```python
from build123d import *

# Parameters (mm, degrees)
SKETCH1_W                        = 125
SKETCH1_H                        = 115
TEST_BASE_POSTION_DEPTH          = 9.215
SKETCH8_R                        = 21.5
FINGER_GEARS_DEPTH               = 5
SKETCH9_R                        = 11
INTERMEDIATE_GEAR_DEPTH          = 5
SKETCH11_R                       = 18
XL320_FINGER_KNUCKLE_MOUNT_DEPTH = 5
SKETCH10_R                       = 15.5
CONNECT_FINGER_HOLES_DEPTH       = 86.424915715
THUMB_MOUNT_HOLES_R              = 2
THUMB_MOUNT_HOLES_M4_DEPTH       = 86.424915715
SKETCH16_R                       = 2
FINGERS_MOUNT_HOLES_M4_DEPTH     = 86.424915715
SKETCH17_R                       = 2.8
CONNECT_HOLES_M6_DEPTH           = 86.424915715
SKETCH18_R                       = 3.75
NUTS_M4_DEPTH                    = 4
SKETCH19_R                       = 5.25
CUT_EXTRUDE5_DEPTH               = 6


with BuildPart() as part:
    # Sketch1 → Test_Base_Postion (new body)
    with BuildSketch(Plane(origin=(0, 0, 0), x_dir=(1, 0, 0), z_dir=(0, 1, 0))):
        Rectangle(SKETCH1_W, SKETCH1_H)
    extrude(amount=TEST_BASE_POSTION_DEPTH)

    # Sketch8 → Finger_Gears (cut)
    with BuildSketch(Plane(origin=(0, 9.215, 0), x_dir=(1, 0, 0), z_dir=(0, 1, 0))):
        with Locations((-32.5, -19)):
            Circle(SKETCH8_R)
        with Locations((-32.5, 19)):
            Circle(SKETCH8_R)
    extrude(amount=-FINGER_GEARS_DEPTH, mode=Mode.SUBTRACT)

    # Sketch9 → Intermediate_Gear (cut)
    with BuildSketch(Plane(origin=(0, 9.215, 0), x_dir=(1, 0, 0), z_dir=(0, 1, 0))):
        with Locations((-8.576859648, -4.450657895)):
            Circle(SKETCH9_R)
    extrude(amount=-INTERMEDIATE_GEAR_DEPTH, mode=Mode.SUBTRACT)

    # Sketch11 → XL320_Finger_Knuckle_Mount (cut)
    with BuildSketch(Plane(origin=(0, 9.215, 0), x_dir=(1, 0, 0), z_dir=(0, 1, 0))):
        with Locations(Location((42, 0, 0), (0, 0, 270))):
            Circle(SKETCH11_R)
    extrude(amount=-XL320_FINGER_KNUCKLE_MOUNT_DEPTH, mode=Mode.SUBTRACT)

    # Sketch10 → Connect_Finger_Holes (cut, through all)
    with BuildSketch(Plane(origin=(0, 9.215, 0), x_dir=(1, 0, 0), z_dir=(0, 1, 0))):
        with Locations(Location((-32.5, 19, 0), (0, 0, 270))):
            Circle(SKETCH10_R)
        with Locations(Location((-32.5, -19, 0), (0, 0, 270))):
            Circle(SKETCH10_R)
        with Locations(Location((42, 0, 0), (0, 0, 270))):
            Circle(SKETCH10_R)
    extrude(amount=-CONNECT_FINGER_HOLES_DEPTH, mode=Mode.SUBTRACT)

    # Thumb_Mount_Holes → Thumb_Mount_Holes_(M4) (cut, through all)
    with BuildSketch(Plane(origin=(0, 9.215, 0), x_dir=(1, 0, 0), z_dir=(0, 1, 0))):
        with Locations(Location((22.5, 45.5, 0), (0, 0, 270))):
            Circle(THUMB_MOUNT_HOLES_R)
        with Locations(Location((42, 52.5, 0), (0, 0, 270))):
            Circle(THUMB_MOUNT_HOLES_R)
        with Locations(Location((48, -24, 0), (0, 0, 270))):
            Circle(THUMB_MOUNT_HOLES_R)
        with Locations(Location((36, -24, 0), (0, 0, 90))):
            Circle(THUMB_MOUNT_HOLES_R)
    extrude(amount=-THUMB_MOUNT_HOLES_M4_DEPTH, mode=Mode.SUBTRACT)

    # Sketch16 → Fingers_Mount_Holes_(M4) (cut, through all)
    with BuildSketch(Plane(origin=(0, 9.215, 0), x_dir=(1, 0, 0), z_dir=(0, 1, 0))):
        with Locations(Location((5.25, 38.5, 0), (0, 0, 270))):
            Circle(SKETCH16_R)
        with Locations(Location((5.25, -38.5, 0), (0, 0, 90))):
            Circle(SKETCH16_R)
    extrude(amount=-FINGERS_MOUNT_HOLES_M4_DEPTH, mode=Mode.SUBTRACT)

    # Sketch17 → Connect_Holes_(M6) (cut, through all)
    with BuildSketch(Plane(origin=(0, 9.215, 0), x_dir=(1, 0, 0), z_dir=(0, 1, 0))):
        with Locations(Location((-52.5, 47.5, 0), (0, 0, 270))):
            Circle(SKETCH17_R)
        with Locations(Location((-52.5, -47.5, 0), (0, 0, 90))):
            Circle(SKETCH17_R)
        with Locations(Location((52.5, -47.5, 0), (0, 0, 270))):
            Circle(SKETCH17_R)
    extrude(amount=-CONNECT_HOLES_M6_DEPTH, mode=Mode.SUBTRACT)

    # Sketch18 → Nuts_(M4) (cut)
    with BuildSketch(Plane.XZ):
        with Locations(Location((5.25, 38.5, 0), (0, 0, 270))):
            Circle(SKETCH18_R)
        with Locations(Location((5.25, -38.5, 0), (0, 0, 270))):
            Circle(SKETCH18_R)
        with Locations(Location((22.5, -45.5, 0), (0, 0, 270))):
            Circle(SKETCH18_R)
        with Locations(Location((42, -52.5, 0), (0, 0, 270))):
            Circle(SKETCH18_R)
        with Locations(Location((36, 24, 0), (0, 0, 270))):
            Circle(SKETCH18_R)
        with Locations(Location((48, 24, 0), (0, 0, 270))):
            Circle(SKETCH18_R)
    extrude(amount=-NUTS_M4_DEPTH, mode=Mode.SUBTRACT)

    # Sketch19 → Cut-Extrude5 (cut)
    with BuildSketch(Plane.XZ):
        with Locations(Location((-52.5, 47.5, 0), (0, 0, 270))):
            Circle(SKETCH19_R)
        with Locations(Location((52.5, 47.5, 0), (0, 0, 270))):
            Circle(SKETCH19_R)
        with Locations(Location((-52.5, -47.5, 0), (0, 0, 270))):
            Circle(SKETCH19_R)
    extrude(amount=-CUT_EXTRUDE5_DEPTH, mode=Mode.SUBTRACT)


solid = part.part
```
The listing builds one solid part. Answer for the finished solid, in the listing's coordinates (mm). A direction names the side the tool comes from. Round coordinates to 2 decimals unless told otherwise and drop trailing zeros. Loops run counter-clockwise (first coordinate to the right, second up) from the corner with the lowest first, then second, coordinate; pieces in that order, holes last.
Q1. Section A-A, the plane y = 2.5 is taken. Count the separate pieces of the cut face and the enclosed holes in it, then the cut area to 3 significant figures.
Q2. Find the intervals of material crossed by line 1 (X direction, y = 2.45, z = 47.5); line 2 (Z direction, x = 43.5, y = 0.5); line 3 (X direction, y = 2, z = 9), in increasing order.
Q3. Given pin 1 Ø6.5 at (x, z) = (-52.5, -47.5) entering from +Y (3 decimals); pin 2 Ø3 at (x, z) = (-52.5, 46) entering from -Y; pin 3 Ø4 at (x, z) = (49, 24) entering from -Y, each flat-ended and moving along its own axis, determine where each tip first touches the part or whether it passes through.
Q4. Section B-B, the plane z = 47.5 is taken. Determine the outline of the cut face in (x, y) (3 decimals), then the cut area to 3 significant figures.
Q5. Which of the six approach directions +Z, -Z, +X, -X, +Y, -Y give full straight-line access (tool end or side, diameter ignored) to faces 3 (the face through (-42.45, 6.75, 38.06)), 4 (the face through (18.84, 1.97, -44.69)), 5 (the face through (40.048, 6.644, -52.934))?
Q6. Section C-C, the plane x = -32.5 is taken. Determine the outline of the cut face in (y, z) (3 decimals).
Q7. Section D-D, the plane z = 24 is taken. Determine the outline of the cut face in (x, y) (3 decimals), then the cut area to 3 significant figures.
Q8. For a pull along Z with two mould halves and no side action, classify faces 1 (the face through (-51.428, 7.63, 44.914)), 2 (the face through (-1, 5, -57.5)) as released by +Z, released by -Z, zero draft, split by the parting line, or undercut.
Completed:
1. separate pieces: 1
1. enclosed holes: 12
1. area: 11,600 mm2
2. line 1: x = -62.5 to -57.75, -47.25 to 47.25, 57.75 to 62.5
2. line 2: z = -57.5 to -55.94, -49.06 to -15.43, 15.43 to 57.5
2. line 3: x = -62.5 to -44.34, -20.66 to 29.38, 54.62 to 62.5
3. pin 1: stops at y = 9.215
3. pin 2: stops at y = 6
3. pin 3: stops at y = 4
4. outline: (-62.5, 0) - (-57.75, 0) - (-57.75, 6) - (-55.3, 6) - (-55.3, 9.215) - (-62.5, 9.215) - close; (-49.7, 6) - (-47.25, 6) - (-47.25, 0) - (47.25, 0) - (47.25, 6) - (49.7, 6) - (49.7, 9.215) - (-49.7, 9.215) - close; (55.3, 6) - (57.75, 6) - (57.75, 0) - (62.5, 0) - (62.5, 9.215) - (55.3, 9.215) - close
4. area: 990 mm2
5. face 3: +Y
5. face 4: -Y
5. face 5: +Y, -Y
6. outline: (0, -57.5) - (9.215, -57.5) - (9.215, -40.5) - (4.215, -40.5) - (4.215, -34.5) - (0, -34.5) - close; (0, -3.5) - (4.215, -3.5) - (4.215, 3.5) - (0, 3.5) - close; (0, 34.5) - (4.215, 34.5) - (4.215, 40.5) - (9.215, 40.5) - (9.215, 57.5) - (0, 57.5) - close
7. outline: (-62.5, 0) - (-47.171, 0) - (-47.171, 4.215) - (-53.411, 4.215) - (-53.411, 9.215) - (-62.5, 9.215) - close; (-17.829, 0) - (32.25, 0) - (32.25, 4) - (34, 4) - (34, 9.215) - (-11.589, 9.215) - (-11.589, 4.215) - (-17.829, 4.215) - close; (38, 4) - (39.75, 4) - (39.75, 0) - (44.25, 0) - (44.25, 4) - (46, 4) - (46, 9.215) - (38, 9.215) - close; (50, 4) - (51.75, 4) - (51.75, 0) - (62.5, 0) - (62.5, 9.215) - (50, 9.215) - close
7. area: 717 mm2
8. face 1: undercut
8. face 2: released by -Z
